```python
from build123d import *

# Parameters (mm, degrees)
SCHIZZO1_R                   = 0.8
ESTRUSIONE_ESTRUSIONE1_DEPTH = 1.8
SCHIZZO2_R                   = 1.5
ESTRUSIONE_ESTRUSIONE2_DEPTH = 6.3
SCHIZZO3_R                   = 1.5
ESTRUSIONE_ESTRUSIONE3_DEPTH = 6.3


with BuildPart() as part:
    # Schizzo1 → Estrusione-Estrusione1 (new body)
    with BuildSketch(Plane.XY):
        with BuildLine():
            Line((-4.9, 4.9), (4.9, 4.9))
            ThreePointArc((4.9, 4.9), (9.8, 0), (4.9, -4.9))
            Line((4.9, -4.9), (-4.9, -4.9))
            ThreePointArc((-4.9, -4.9), (-9.8, 0), (-4.9, 4.9))
        make_face()
        with Locations((4.4, 0)):
            Circle(SCHIZZO1_R, mode=Mode.SUBTRACT)
    extrude(amount=ESTRUSIONE_ESTRUSIONE1_DEPTH)

    # Schizzo2 → Estrusione-Estrusione2 (add)
    with BuildSketch(Plane.XY.offset(1.8)):
        with Locations((-6.3, 0)):
            Circle(SCHIZZO2_R)
    extrude(amount=ESTRUSIONE_ESTRUSIONE2_DEPTH)

    # Schizzo3 → Estrusione-Estrusione3 (add)
    with BuildSketch(Plane.XY.offset(1.8)):
        with Locations((6.8, 0)):
            Circle(SCHIZZO3_R)
    extrude(amount=ESTRUSIONE_ESTRUSIONE3_DEPTH)


solid = part.part
```
The model under review builds one solid part; all positions refer to its coordinate system, in mm. A direction names the side the tool comes from. Coordinates: 2 decimals unless noted, no trailing zeros. Write each loop counter-clockwise with the first axis right and the second up, starting at its lowest first coordinate (ties: lowest second). Pieces come first, ordered by that corner, then holes. Notation, with made-up numbers: (61, -29) -> (90, -29) arc R27 ccw to (90, 8) -> close; hole circle Ø1 at (54.25, 85.25). An arc over 180 degrees is marked (long way). One line per item, written item: value. Start each with the question number.
Q1. Add section D-D, the plane x = -6. Give the boundary of the cut face in (y, z).
Q2. Add section B-B, the plane y = 0. Give the boundary of the cut face in (x, z), then the cut area to 3 significant figures.
Q3. To check wall thickness, follow probe 1 along Y at (x, z) = (4.4, 0.75); probe 2 along Z at (x, y) = (-5, 2.5); probe 3 along X at (y, z) = (-0.5, 7.5). State the ranges of each line that lie inside material, in increasing order.
Q4. Add section A-A, the plane x = 4.4. Give the boundary of the cut face in (y, z).
Q5. Clearance check with flat-ended pins moving along their axes: P1, Ø1.5, axis at y = -1.5, z = 5.5, coming from the +X side; P2, Ø4, axis at x = -7.5, z = 2.5, coming from the +Y side. State where each tip first meets the part, or that it passes through.
Q6. Add section C-C, the plane z = 3.25. Give the boundary of the cut face in (x, y), then the cut area to 3 significant figures.
Q7. For faces 1 (the face through (5.3, 0.07, 4.91)), 2 (the face through (7, 0, 8.1)), list the 3-axis set-ups (+Z, -Z, +X, -X, +Y, -Y) from which the entire face can be reached by the end or side of a thin tool; tool diameter is ignored.
Q8. The part is to be moulded in two halves that separate along Y. For faces 3 (the face through (-4.87, 0.45, 4.91)), 4 (the face through (0, 4.9, 1)), 5 (the face through (5.163, 0.24, 0.887)), 6 (the face through (0, -4.9, 1)), say which applies: +Y half, -Y half, draft (parallel to the pull), parting line (faces both ways), or undercut.
Response:
1. outline: (-4.77, 0) -> (4.77, 0) -> (4.77, 1.8) -> (1.47, 1.8) -> (1.47, 8.1) -> (-1.47, 8.1) -> (-1.47, 1.8) -> (-4.77, 1.8) -> close
2. outline: (-9.8, 0) -> (3.6, 0) -> (3.6, 1.8) -> (-4.8, 1.8) -> (-4.8, 8.1) -> (-7.8, 8.1) -> (-7.8, 1.8) -> (-9.8, 1.8) -> close; (5.2, 0) -> (9.8, 0) -> (9.8, 1.8) -> (8.3, 1.8) -> (8.3, 8.1) -> (5.3, 8.1) -> (5.3, 1.8) -> (5.2, 1.8) -> close
2. area: 70.2 mm²
3. probe 1: -4.9 to -0.8, 0.8 to 4.9
3. probe 2: 0 to 1.8
3. probe 3: -7.71 to -4.89, 5.39 to 8.21
4. outline: (-4.9, 0) -> (-0.8, 0) -> (-0.8, 1.8) -> (-4.9, 1.8) -> close; (0.8, 0) -> (4.9, 0) -> (4.9, 1.8) -> (0.8, 1.8) -> close
5. P1: x = 8.1
5. P2: y = 4.85
6. outline: circle Ø3 at (-6.3, 0); circle Ø3 at (6.8, 0)
6. area: 14.1 mm²
7. face 1: +Z
7. face 2: +Z, +X, -X, +Y, -Y
8. face 3: parting line
8. face 4: +Y half
8. face 5: undercut
8. face 6: -Y half
